Can you work these out from the drawing? Everything is in mm from the part's minimum corner. A direction names the side the tool comes from. Coordinates: 2 decimals unless noted, no trailing zeros. Order: outer loops, then holes, each group sorted by start corner. A loop starts at its lowest first (then second) coordinate and runs counter-clockwise, first axis right, second up. Notation, with made-up numbers: (61, -33.5) - (95, -33.5) arc R11 cw to (95, -18.5) - close; hole circle Ø6 at (-30.5, -19). An arc over 180 degrees is marked (long way). Answer as CSV lines item,"result". Start each with the question number.
Q1. I need wall thicknesses on line 1 (Y direction, x = 11, z = 4); line 2 (X direction, y = 27.5, z = 5); line 3 (X direction, y = 5.5, z = 5). Which ranges of each line are inside material? Lowest first, please.
Q2. For the marked faces 4, 5, 6 and 7, which set-ups out of +Z, -Z, +X, -X, +Y, -Y let a thin tool reach every point of the face, with its end or its side?
Q3. Suppose I cut it at D-D (z = 6). Please give me the cut outline in (x, y), then the cut area to 3 significant figures.
Q4. Thinking about a two-plate mould opening in Y: for the marked faces 1, 2 and 3, which applies, released by +Y, released by -Y, zero draft, split by the parting line, or undercut?
Q5. Suppose I cut it at B-B (z = 9.75). Please give me the cut outline in (x, y).
Q6. For pin 1 Ø2.5 at (y, z) = (3, 6.5) entering from -X; pin 2 Ø3 at (x, y) = (14, 24.5) entering from -Z; pin 3 Ø2 at (x, y) = (12, 18.5) entering from -Z; pin 4 Ø1.6 at (x, z) = (12, 4.5) entering from +Y, each with a flat end and sliding along its axis, tell me the tip position at first contact or that it passes through.
Q7. Suppose I cut it at A-A (y = 18.5). Please give me the cut outline in (x, z), then the cut area to 3 significant figures.
Q8. Suppose I cut it at C-C (x = 1). Please give me the cut outline in (y, z), then the cut area to 3 significant figures.
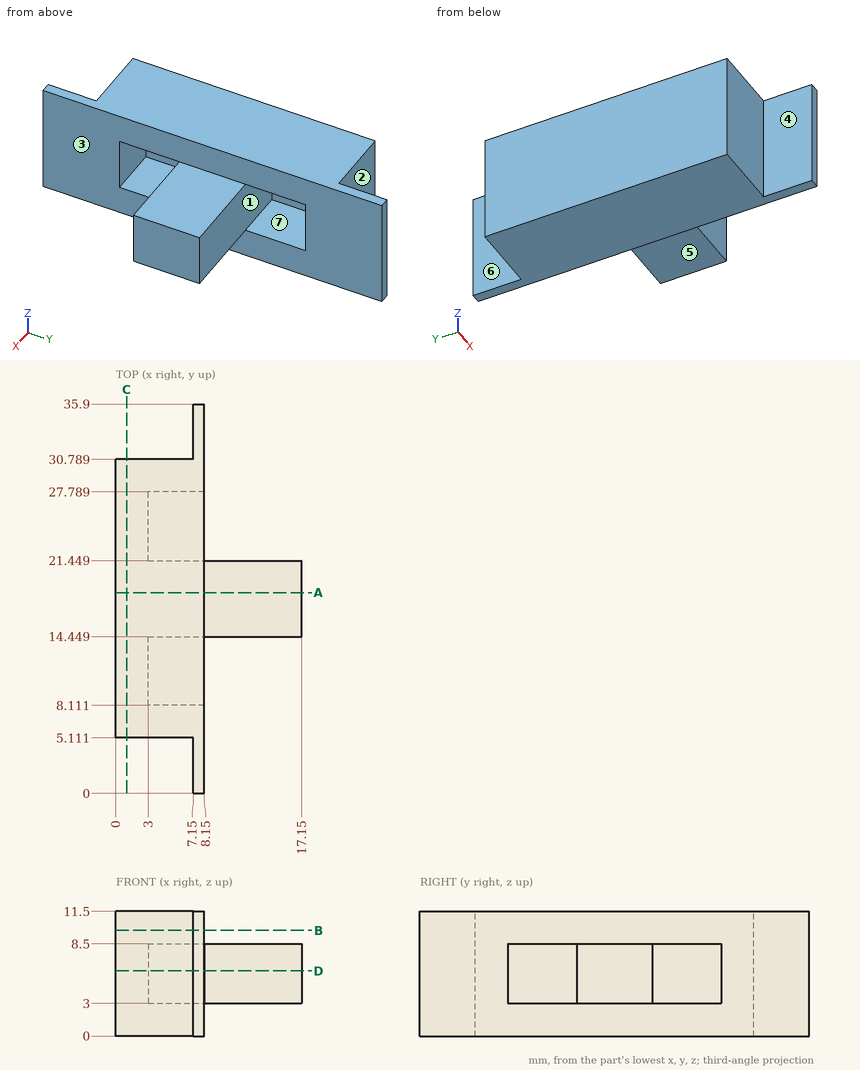
Here are the results:
1,line 1,"y = 14.45 to 21.45"
1,line 2,"x = 0 to 3"
1,line 3,"x = 0 to 8.15"
2,face 4,"+Z, -Z, -X, -Y"
2,face 5,"-Z, +X, +Y, -Y"
2,face 6,"+Z, -Z, -X, +Y"
2,face 7,"+X"
3,outline,"(0, 5.11) - (7.15, 5.11) - (7.15, 0) - (8.15, 0) - (8.15, 8.11) - (3, 8.11) - (3, 14.45) - (17.15, 14.45) - (17.15, 21.45) - (3, 21.45) - (3, 27.79) - (8.15, 27.79) - (8.15, 35.9) - (7.15, 35.9) - (7.15, 30.79) - (0, 30.79) - close"
3,area,"217 mm²"
4,face 1,"undercut"
4,face 2,"released by +Y"
4,face 3,"zero draft"
5,outline,"(0, 5.11) - (7.15, 5.11) - (7.15, 0) - (8.15, 0) - (8.15, 35.9) - (7.15, 35.9) - (7.15, 30.79) - (0, 30.79) - close"
6,pin 1,"stops at x = 7.15"
6,pin 2,"passes through"
6,pin 3,"stops at z = 3"
6,pin 4,"stops at y = 21.45"
7,outline,"(0, 0) - (8.15, 0) - (8.15, 3) - (17.15, 3) - (17.15, 8.5) - (8.15, 8.5) - (8.15, 11.5) - (0, 11.5) - close"
7,area,"143 mm²"
8,outline,"(5.11, 0) - (30.79, 0) - (30.79, 11.5) - (5.11, 11.5) - close"
8,area,"295 mm²"
